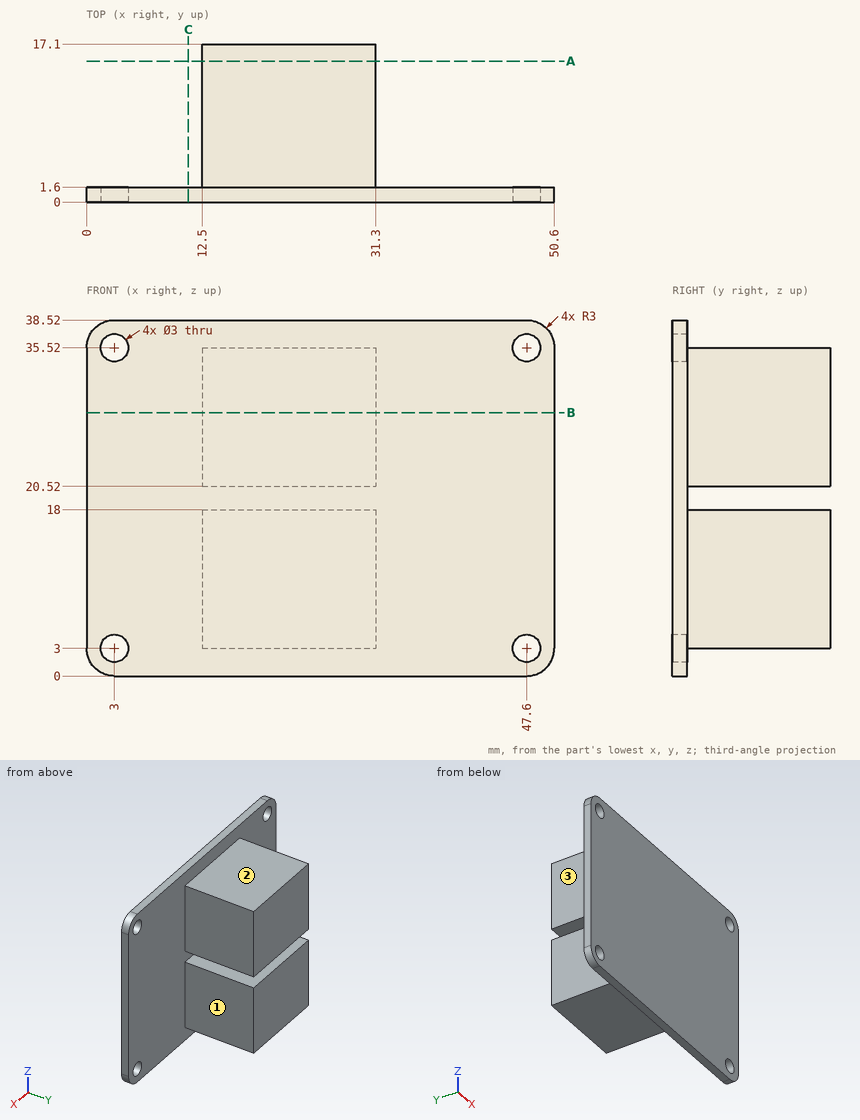
Can you work these out from the drawing? Everything is in mm from the part's minimum corner. A direction names the side the tool comes from. Round coordinates to 2 decimals unless told otherwise and drop trailing zeros. Loops run counter-clockwise (first coordinate to the right, second up) from the corner with the lowest first, then second, coordinate; pieces in that order, holes last. Notation, with made-up numbers: (-19.75, 65) -> (32.25, 65) arc R14 ccw to (32.25, 72) -> close; hole circle Ø8 at (83, -38.5). An arc over 180 degrees is marked (long way). Answer in a Markdown table with one row per item.
Item 1: Suppose I cut it at A-A, the plane y = 15.25. List the corners of the cut face in (x, z) for me.
Answer block:
| item | result |
|---|---|
| outline | (12.5, 3) -> (31.3, 3) -> (31.3, 18) -> (12.5, 18) -> close; (12.5, 20.52) -> (31.3, 20.52) -> (31.3, 35.52) -> (12.5, 35.52) -> close |
Item 2: Suppose I cut it at C-C, the plane x = 11. List the corners of the cut face in (y, z) for me, plus the area to 3 significant figures.
Answer block:
| item | result |
|---|---|
| outline | (0, 0) -> (1.6, 0) -> (1.6, 38.52) -> (0, 38.52) -> close |
| area | 61.6 mm² |
Item 3: Will these pins go through, and if not, where does the flat tip stop? P1, Ø4.5, axis at y = 11.5, z = 27.5, coming from the +X side; P2, Ø3, axis at x = 5.5, z = 6.5, coming from the +Y side; P3, Ø2.5, axis at x = 3, z = 3, coming from the -Y side; P4, Ø8, axis at x = 19, y = 6, coming from the +Z side.
Answer block:
| item | result |
|---|---|
| P1 | x = 31.3 |
| P2 | y = 1.6 |
| P3 | through |
| P4 | z = 35.52 |
Item 4: Suppose I cut it at B-B, the plane z = 28.5. List the corners of the cut face in (x, y) for me.
Answer block:
| item | result |
|---|---|
| outline | (0, 0) -> (50.6, 0) -> (50.6, 1.6) -> (31.3, 1.6) -> (31.3, 17.1) -> (12.5, 17.1) -> (12.5, 1.6) -> (0, 1.6) -> close |
Item 5: On a 3-axis mill with a long thin cutter (end or side, diameter ignored), from which of +Z, -Z, +X, -X, +Y, -Y can I reach the whole of each face in a straight line? I mean the marked faces 1, 2 and 3. Say none if no direction works.
Answer block:
| item | result |
|---|---|
| face 1 | +Z, -Z, +X, +Y |
| face 2 | +Z, +X, -X, +Y |
| face 3 | +Z, -Z, -X, +Y |
Item 6: If I drill on probe 1 along X at (y, z) = (1.05, 35.52); probe 2 along Z at (x, y) = (21.5, 12.5); probe 3 along Y at (x, z) = (6.5, 16), over which ranges is the centre line in solid material (lowest first)?
Answer block:
| item | result |
|---|---|
| probe 1 | 0 to 1.5, 4.5 to 46.1, 49.1 to 50.6 |
| probe 2 | 3 to 18, 20.52 to 35.52 |
| probe 3 | 0 to 1.6 |
